from build123d import *

# Parameters (mm, degrees)
SKETCH2_R                               = 2.4
BOSS_EXTRUDE1_DEPTH                     = 35.814
CUT_EXTRUDE1_DEPTH                      = 8.45076
CBORE_FOR_M5_HEX_HEAD_BOLT1_D           = 5.5
CBORE_FOR_M5_HEX_HEAD_BOLT1_CBORE_D     = 12.24
CBORE_FOR_M5_HEX_HEAD_BOLT1_CBORE_DEPTH = 3.58
BOSS_EXTRUDE2_DEPTH                     = 12
CBORE_FOR_M5_HEX_HEAD_BOLT2_D           = 5.5
CBORE_FOR_M5_HEX_HEAD_BOLT2_DEPTH       = 12
CBORE_FOR_M5_HEX_HEAD_BOLT2_CBORE_D     = 12.24
CBORE_FOR_M5_HEX_HEAD_BOLT2_CBORE_DEPTH = 3.58
CUT_EXTRUDE2_REACH                      = 106.459
SKETCH11_R                              = 2.4


with BuildPart() as part:
    # Sketch2 → Boss-Extrude1 (new body)
    with BuildSketch(Plane(origin=(0, 0, 0), x_dir=(1, 0, 0), z_dir=(0, 1, 0))):
        Polygon((79.858578644, 45.6), (79.858578644, 11.5), (39.5, 11.5), (39.4, 19.95075985), (34.265987805, 23.9), (33.603154542, 24.5), (23.866312437, 31.9), (7.8, 32), (7.8, 35.6), (0, 35.6), (0, 32), (-0.1, 27.6), (-9.6, 27.6), (-9.6, 45.6), align=None)
        with Locations((67.9, 16)):
            Circle(SKETCH2_R, mode=Mode.SUBTRACT)
        with Locations((51.9, 16)):
            Circle(SKETCH2_R, mode=Mode.SUBTRACT)
        with Locations((59.9, 16)):
            Circle(SKETCH2_R, mode=Mode.SUBTRACT)
    extrude(amount=BOSS_EXTRUDE1_DEPTH)

    # Sketch4 → Cut-Extrude1 (cut)
    with BuildSketch(Plane.XY.offset(-11.5)):
        Polygon((67.9, 22.307), (51.9, 22.307), (47.8, 22.307), (47.8, 13.507), (51.9, 13.507), (67.9, 13.507), (72, 13.507), (72, 22.307), align=None)
    extrude(amount=-CUT_EXTRUDE1_DEPTH, mode=Mode.SUBTRACT)

    # CBORE for M5 Hex Head Bolt1 (through all)
    with Locations(Plane(origin=(0.199468966, 0, -32.047307253), x_dir=(0.99998063, 0, 0.006224083), z_dir=(-0.006224083, 0, 0.99998063))):
        with Locations((15.578271559, 27.314), (15.600678258, 8.5)):
            CounterBoreHole(CBORE_FOR_M5_HEX_HEAD_BOLT1_D / 2, CBORE_FOR_M5_HEX_HEAD_BOLT1_CBORE_D / 2, CBORE_FOR_M5_HEX_HEAD_BOLT1_CBORE_DEPTH)

    # Sketch8 → Boss-Extrude2 (add)
    with BuildSketch(Plane(origin=(0, 0, -45.6), x_dir=(-1, 0, 0), z_dir=(0, 0, -1))):
        Polygon((-79.858578644, 35.814), (-94.858578644, 25.407), (-94.858578644, 10.407), (-79.858578644, 0), align=None)
    extrude(amount=-BOSS_EXTRUDE2_DEPTH)

    # CBORE for M5 Hex Head Bolt2
    with Locations(Plane.XY.offset(-33.6)):
        with Locations((87.358578644, 17.907)):
            CounterBoreHole(CBORE_FOR_M5_HEX_HEAD_BOLT2_D / 2, CBORE_FOR_M5_HEX_HEAD_BOLT2_CBORE_D / 2, CBORE_FOR_M5_HEX_HEAD_BOLT2_CBORE_DEPTH, depth=CBORE_FOR_M5_HEX_HEAD_BOLT2_DEPTH)

    # Sketch11 → Cut-Extrude2 (cut, up to next)
    with BuildSketch(Plane.ZY.offset(9.6), mode=Mode.PRIVATE) as cut_extrude2_sk1:
        with Locations((-32, 25.814)):
            Circle(SKETCH11_R)
    cut_extrude2_tool1 = extrude(cut_extrude2_sk1.sketch, amount=-CUT_EXTRUDE2_REACH, mode=Mode.PRIVATE) & part.part
    add(cut_extrude2_tool1.solids().sort_by_distance((-9.6, 25.814, -32))[0], mode=Mode.SUBTRACT)
    # Sketch11 → Cut-Extrude2 (cut, up to next)
    with BuildSketch(Plane.ZY.offset(9.6), mode=Mode.PRIVATE) as cut_extrude2_sk2:
        with Locations((-32, 17.814)):
            Circle(SKETCH11_R)
    cut_extrude2_tool2 = extrude(cut_extrude2_sk2.sketch, amount=-CUT_EXTRUDE2_REACH, mode=Mode.PRIVATE) & part.part
    add(cut_extrude2_tool2.solids().sort_by_distance((-9.6, 17.814, -32))[0], mode=Mode.SUBTRACT)
    # Sketch11 → Cut-Extrude2 (cut, up to next)
    with BuildSketch(Plane.ZY.offset(9.6), mode=Mode.PRIVATE) as cut_extrude2_sk3:
        with Locations((-32, 9.814)):
            Circle(SKETCH11_R)
    cut_extrude2_tool3 = extrude(cut_extrude2_sk3.sketch, amount=-CUT_EXTRUDE2_REACH, mode=Mode.PRIVATE) & part.part
    add(cut_extrude2_tool3.solids().sort_by_distance((-9.6, 9.814, -32))[0], mode=Mode.SUBTRACT)


solid = part.part
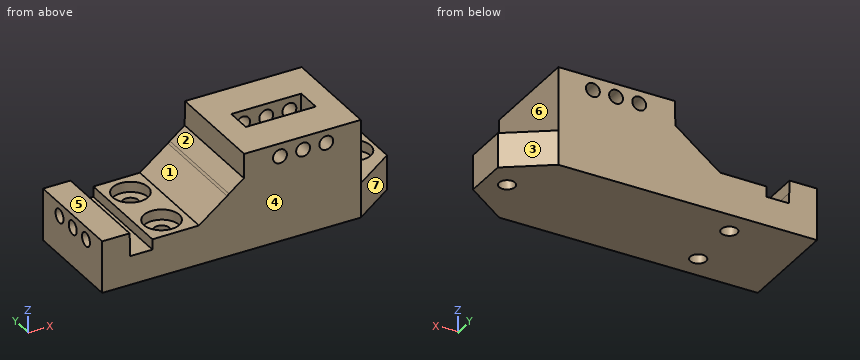
Check sheet for the modelled part. Datum: model origin and axes. Units: mm. Face numbers are marked on the shaded views. A direction names the side the tool comes from. Round coordinates to 2 decimals unless told otherwise and drop trailing zeros. Order: outer loops, then holes, each group sorted by start corner. A loop starts at its lowest first (then second) coordinate and runs counter-clockwise, first axis right, second up.
(1) Access from +Z, -Z, +X, -X, +Y, -Y to the whole of each face (thin tool, end or side, straight path). Record for the marked faces 5, 6 and 7.
(2) Go/stop test with flat-tipped pins: P1, Ø7, axis at x = 87.36, y = 17.91, coming from the +Z side; P2, Ø4.5, axis at x = 67.9, z = -16, coming from the -Y side; P3, Ø4.5, axis at x = 88.5, y = 23.5, coming from the +Z side; P4, Ø4, axis at y = 25.814, z = -32, coming from the -X side. Record where each tip stops, or that it passes through.
(3) Cross-section at C-C, the plane z = -15. State how many separate pieces and enclosed holes the cut face has, and give its area (3 significant figures).
(4) Cross-section at B-B, the plane y = 32. Enter the section's corners in (x, z).
(5) Scan lines: probe 1 along Y at (x, z) = (-3, -32); probe 2 along Y at (x, z) = (15.5, -33); probe 3 along X at (y, z) = (6, -16). Record each from-to range of solid material in increasing order.
(6) Cross-section at D-D, the plane x = 86. Enter the section's corners in (y, z), and give its area (3 significant figures).
(7) Draft check along X on the marked faces 1, 2, 3 and 4. Enter one of: pulls with the +X half, pulls with the -X half, needs draft (parallel to the pull), parting line crosses it, or undercut.
(8) Cross-section at A-A, the plane x = 59.9. Enter the section's corners in (y, z).
Check sheet entries:
1. face 5: +Z, -X, +Y, -Y
1. face 6: +Z, +X, +Y, -Y
1. face 7: +Z, -Z, +X, -Y
2. P1: stops at z = -37.18
2. P2: passes through
2. P3: stops at z = -33.6
2. P4: stops at x = 7.8
3. separate pieces: 6
3. enclosed holes: 0
3. area: 880 mm2
4. outline: (-9.6, -45.6) - (85.36, -45.6) - (85.36, -33.6) - (79.86, -33.6) - (79.86, -11.5) - (39.5, -11.5) - (39.4, -19.95) - (34.27, -23.9) - (33.6, -24.5) - (23.87, -31.9) - (19.71, -31.93) - (19.74, -35.51) - (11.86, -35.55) - (11.84, -31.97) - (7.8, -32) - (7.8, -35.6) - (0, -35.6) - (0, -32) - (-0.1, -27.6) - (-9.6, -27.6) - close; hole circle Ø4.8 at (51.9, -16); hole circle Ø4.8 at (59.9, -16); hole circle Ø4.8 at (67.9, -16)
5. probe 1: y = 0 to 7.41, 12.21 to 15.41, 20.21 to 23.41, 28.21 to 35.81
5. probe 2: y = 0 to 2.39, 14.61 to 21.2, 33.43 to 35.81
5. probe 3: x = 39.45 to 49.5, 54.3 to 57.5, 62.3 to 65.5, 70.3 to 79.86
6. outline: (4.26, -45.6) - (15.52, -45.6) - (15.52, -37.18) - (11.94, -37.18) - (11.94, -33.6) - (4.26, -33.6) - close; (20.3, -45.6) - (31.55, -45.6) - (31.55, -33.6) - (23.87, -33.6) - (23.87, -37.18) - (20.3, -37.18) - close
6. area: 245 mm2
7. face 1: undercut
7. face 2: pulls with the -X half
7. face 3: pulls with the +X half
7. face 4: needs draft
8. outline: (0, -45.6) - (35.81, -45.6) - (35.81, -18.4) - (22.31, -18.4) - (22.31, -19.95) - (13.51, -19.95) - (13.51, -18.4) - (0, -18.4) - close; (0, -13.6) - (13.51, -13.6) - (13.51, -11.5) - (0, -11.5) - close; (22.31, -13.6) - (35.81, -13.6) - (35.81, -11.5) - (22.31, -11.5) - close
